Geometry check sheet. Reference: the model listing, model coordinates, mm. A direction names the side the tool comes from. Round coordinates to 2 decimals unless told otherwise and drop trailing zeros. Order: outer loops, then holes, each group sorted by start corner. A loop starts at its lowest first (then second) coordinate and runs counter-clockwise, first axis right, second up.
(1) Sectioned sample at B-B (z = 19.75). Record the boundary of the cut face in (x, y).
(2) Sectioned sample at A-A (x = -44). Record the boundary of the cut face in (y, z), plus the area to 3 significant figures.
(3) Go/stop test with flat-tipped pins: pin 1 (1.5 mm diameter, centred on x = 0.5, z = 2, fed in from +Y); pin 2 (8 mm diameter, centred on x = -263.5, z = 20.5, fed in from +Y); pin 3 (3.5 mm diameter, centred on y = 39, z = 1.5, fed in from -X). Record where each tip stops, or that it passes through.
(4) Material ranges on line 1 along Y through (x, z) = (553, 27.5); line 2 along Y through (x, z) = (-643, 2.75), recorded low to high.
(5) Set-up check for faces 1 (the face through (10, 3, 18)), 2 (the face through (-10, 28, 0)): record each of +Z, -Z, +X, -X, +Y, -Y from which the full face is reachable in a straight line by a thin tool's end or side.
Autodesk Inventor part; units mm, degrees
ref_plane "YZ Plane" through (0, 0, 0) normal (1, 0, 0) x (0, 1, 0)
ref_plane "XZ Plane" through (0, 0, 0) normal (0, 1, 0) x (-1, 0, 0)
ref_plane "XY Plane" through (0, 0, 0) normal (0, 0, 1) x (1, 0, 0)
sketch "Sketch1" plane through (0, 0, 0) normal (0, 0, 1) x (1, 0, 0)
  line L0 (-750, 50) -> (750, 50)
  line L1 (750, 50) -> (750, 0)
  line L2 (750, 0) -> (-750, 0)
  line L3 (-750, 0) -> (-750, 50)
  point P0 (0, 0)
  point P1 (0, 0)
  dimension "d0" = 1500
  dimension "d1" = 50
extrude "Plate1" add sketch "Sketch1" along normal blind 3
sketch "Sketch2" plane through (750, 3, 0) normal (0, -1, 0) x (1, 0, 0)
  line L0 (-1500, 0) -> (0, 0)
  line L1 (0, 0) -> (0, 30)
  line L2 (0, 30) -> (-1500, 30)
  line L3 (-1500, 30) -> (-1500, 0)
edge flange "Flange1" height 30 angle 90 thickness 3 bend radius 3 thickness toward (0, -1, 0) relief tear relief width 3 relief depth 1.5 edges at (0, 0, 3) wall of the first edge with corners at (-750, 3, 0) (750, 3, 0) (750, 3, 30) (-750, 3, 30)
bend "Bend1"
corner "Corner1"
sketch "Sketch5" plane through (0, 0, 0) normal (0, 0, -1) x (-1, 0, 0)
  line L0 (750, 50) -> (-750, 50)
  line L1 (497, 50) -> (497, 31)
  line L2 (497, 31) -> (500, 31)
  line L3 (500, 31) -> (500, 50) construction
  line L4 (750, 0) -> (-750, 0)
  line L5 (500, 31) -> (503, 31)
  line L6 (503, 31) -> (503, 50)
  point P0 (0, 0)
  dimension "d18" = 3
  dimension "d19" = 250
  dimension "d20" = 31
  dimension "d27" = 3
extrude "Extrusion1" cut sketch "Sketch5" against normal through all
pattern_linear "Rectangular Pattern1" count 3 spacing 500 along (1, 0, 0) of "Extrusion1"
sketch "Sketch6" plane through (0, 0, 0) normal (0, 0, -1) x (-1, 0, 0)
  line L0 (-750, 50) -> (-750, 6)
  circle A0 centre (-750, 50) radius 15
  line L1 (-750, 50) -> (750, 50)
  point P0 (0, 0)
  point P1 (-503, 50)
  point P2 (-735, 50)
  point P3 (-750, 35)
  dimension "d24" = 30
extrude "Extrusion2" cut sketch "Sketch6" against normal through all contours L1 A0 L0 picked at (-740.1254, 48.8874)
mirror "Mirror1" about plane through (0, 0, 0) normal (1, 0, 0) of "Extrusion2"
equation "\"d1\" = Стрингер_1"
equation "\"d18\" = Thickness"
equation "\"d27\" = d18"
equation "\"d2\" = Thickness"
equation "\"d3\" = BendReliefWidth"
equation "\"d4\" = BendReliefDepth"
equation "\"d5\" = MinimumRemnant"
equation "\"d6\" = TransitionRadius"
equation "\"d9\" = BendRadius"
equation "\"d10\" = CornerReliefSize"
equation "\"d11\" = GapSize"
equation "\"d12\" = JacobiRadiusSize"
equation "\"BendRadius\" = Thickness"
equation "\"BendReliefWidth\" = Thickness"
equation "\"BendReliefDepth\" = 0.5 * Thickness"
equation "\"CornerReliefSize\" = 4 * Thickness"
equation "\"MinimumRemnant\" = 2 * Thickness"
equation "\"TransitionRadius\" = BendRadius"
equation "\"JacobiRadiusSize\" = BendRadius"
equation "\"GapSize\" = Thickness"
equation "\"qqqqqq\" = 67.35706"
properties part number "МОО 051 стрингер спина 12"
Answer below:
1. outline: (-750, 0) - (750, 0) - (750, 3) - (-750, 3) - close
2. outline: (0, 6) arc R6 ccw to (6, 0) - (50, 0) - (50, 3) - (6, 3) arc R3 cw to (3, 6) - (3, 30) - (0, 30) - close
2. area: 225 mm2
3. pin 1: stops at y = 31
3. pin 2: stops at y = 3
3. pin 3: stops at x = -742.1
4. line 1: y = 0 to 3
4. line 2: y = 0.96 to 50
5. face 1: +Z, +X, -X, +Y
5. face 2: -Z, +X, -X, +Y, -Y
